```python
from build123d import *

# Parameters (mm, degrees)
ESBO_O1_W                = 40
ESBO_O1_H                = 30
RESSALTO_EXTRUS_O1_DEPTH = 10
RESSALTO_EXTRUS_O2_DEPTH = 5
RESSALTO_EXTRUS_O3_DEPTH = 20
ESBO_O4_W                = 10
ESBO_O4_H                = 10
CORTE_EXTRUS_O1_DEPTH    = 41
ESBO_O5_R                = 5
CORTE_EXTRUS_O2_DEPTH    = 16


with BuildPart() as part:
    # Esboço1 → Ressalto-extrusão1 (new body)
    with BuildSketch(Plane(origin=(0, 0, 0), x_dir=(1, 0, 0), z_dir=(0, 1, 0))):
        Rectangle(ESBO_O1_W, ESBO_O1_H)
    extrude(amount=RESSALTO_EXTRUS_O1_DEPTH)

    # Esboço2 → Ressalto-extrusão2 (add)
    with BuildSketch(Plane(origin=(0, 10, 0), x_dir=(1, 0, 0), z_dir=(0, 1, 0))):
        with BuildLine():
            Line((20, 10), (20, -10))
            Line((20, -10), (-5, -10))
            ThreePointArc((-5, -10), (-15, 0), (-5, 10))
            Line((-5, 10), (20, 10))
        make_face()
    extrude(amount=RESSALTO_EXTRUS_O2_DEPTH)

    # Esboço3 → Ressalto-extrusão3 (add)
    with BuildSketch(Plane.XY.offset(10)):
        Polygon((20, 15), (5, 15), (15, 30), (20, 30), align=None)
    extrude(amount=-RESSALTO_EXTRUS_O3_DEPTH)

    # Esboço4 → Corte-extrusão1 (cut, through all)
    with BuildSketch(Plane(origin=(20, 0, 0), x_dir=(0, 0, -1), z_dir=(1, 0, 0))):
        with Locations((0, 25)):
            Rectangle(ESBO_O4_W, ESBO_O4_H)
    extrude(amount=-CORTE_EXTRUS_O1_DEPTH, mode=Mode.SUBTRACT)

    # Esboço5 → Corte-extrusão2 (cut, through all)
    with BuildSketch(Plane(origin=(0, 15, 0), x_dir=(1, 0, 0), z_dir=(0, 1, 0))):
        with Locations((-5, 0)):
            Circle(ESBO_O5_R)
    extrude(amount=-CORTE_EXTRUS_O2_DEPTH, mode=Mode.SUBTRACT)


solid = part.part
```
For this review, take the finished solid that the model builds, in its own axes (mm). A direction names the side the tool comes from. Give positions to 0.01 mm unless a question says otherwise; leave off trailing zeros. Order: outer loops, then holes, each group sorted by start corner. A loop starts at its lowest first (then second) coordinate and runs counter-clockwise, first axis right, second up.
1) Take a section at C-C (x = 2). Give the boundary of the cut face in (y, z), then the cut area to 3 significant figures.
2) Take a section at A-A (z = 0). Give the boundary of the cut face in (x, y).
3) The part is to be moulded in two halves that separate along Z. For faces 6 (the face through (-15, 12, 0)), 7 (the face through (16, 24, 5)), 8 (the face through (17, 30, 8)), say which applies: released by +Z, released by -Z, zero draft, split by the parting line, or undercut.
4) Wall thickness on line 1 (Z direction, x = -5, y = 7.75); line 2 (Z direction, x = -5, y = 11.75); line 3 (X direction, y = 3.5, z = 0): over which ranges is each line inside the solid? List them lowest first.
5) For faces 1 (the face through (10, 18, 10)), 2 (the face through (10, 18, -10)), 3 (the face through (0, 15, 2)), 4 (the face through (16, 24, -5)), 5 (the face through (-4.7, 10, -10.2)), list the 3-axis set-ups (+Z, -Z, +X, -X, +Y, -Y) from which the entire face can be reached by the end or side of a thin tool; tool diameter is ignored.
6) Take a section at B-B (y = 26.5). Give the boundary of the cut face in (x, z).
7) Take a section at D-D (y = 7.75). Give the boundary of the cut face in (x, z).
8) Insertion check: pin 1 (5 mm diameter, centred on x = 8.5, z = -5.5, fed in from -Y); pin 2 (9 mm diameter, centred on x = -5, z = 0, fed in from +Y); pin 3 (1 mm diameter, centred on x = 8.5, y = 16.5, fed in from +Z); pin 4 (1 mm diameter, centred on y = 17, z = -4.5, fed in from -X). Each pin has a flat end and moves straight along its axis. Give the tip position at first contact, or say it passes through.
Derived:
1. outline: (0, -15) - (10, -15) - (10, -10) - (15, -10) - (15, 10) - (10, 10) - (10, 15) - (0, 15) - close
1. area: 400 mm2
2. outline: (-20, 0) - (-10, 0) - (-10, 15) - (-15, 15) - (-15, 10) - (-20, 10) - close; (0, 0) - (20, 0) - (20, 20) - (8.33, 20) - (5, 15) - (0, 15) - close
3. face 6: split by the parting line
3. face 7: undercut
3. face 8: zero draft
4. line 1: z = -15 to -5, 5 to 15
4. line 2: z = -10 to -5, 5 to 10
4. line 3: x = -20 to -10, 0 to 20
5. face 1: +Z, +X, -X, +Y
5. face 2: -Z, +X, -X, +Y
5. face 3: +Z, -Z, -X, +Y
5. face 4: +X, -X, +Y
5. face 5: -X, +Y
6. outline: (12.67, -10) - (20, -10) - (20, -5) - (12.67, -5) - close; (12.67, 5) - (20, 5) - (20, 10) - (12.67, 10) - close
7. outline: (-20, -15) - (20, -15) - (20, 15) - (-20, 15) - close; hole circle Ø10 at (-5, 0)
8. pin 1: stops at y = 0
8. pin 2: passes through
8. pin 3: stops at z = 10
8. pin 4: stops at x = 6
